Here's the drawing with two shaded views (mm, measured from the low corner). I have some questions. A direction names the side the tool comes from. Coordinates: 2 decimals unless noted, no trailing zeros. Write each loop counter-clockwise with the first axis right and the second up, starting at its lowest first coordinate (ties: lowest second). Pieces come first, ordered by that corner, then holes.
Item 1: If I drill on line 1 (Z direction, x = 100.5, y = 17.5); line 2 (Y direction, x = 9.5, z = 70), over which ranges is the centre line in solid material (lowest first)?
Item 2: For the marked faces 1 and 2, which set-ups out of +Z, -Z, +X, -X, +Y, -Y let a thin tool reach every point of the face, with its end or its side?
Item 3: If we section it at B-B (x = 35): Please give me the cut outline in (y, z).
Item 4: If we section it at C-C (z = 157.5): Please give me the cut outline in (x, y).
Item 5: If we section it at A-A (y = 26): Please give me the cut outline in (x, z), then the cut area to 3 significant figures.
Item 6: I'm going to push a flat-ended pin straight in: pin 1 Ø8 at (x, z) = (26, 38.5) entering from -Y. Where does the tip first touch, or does it pass through?
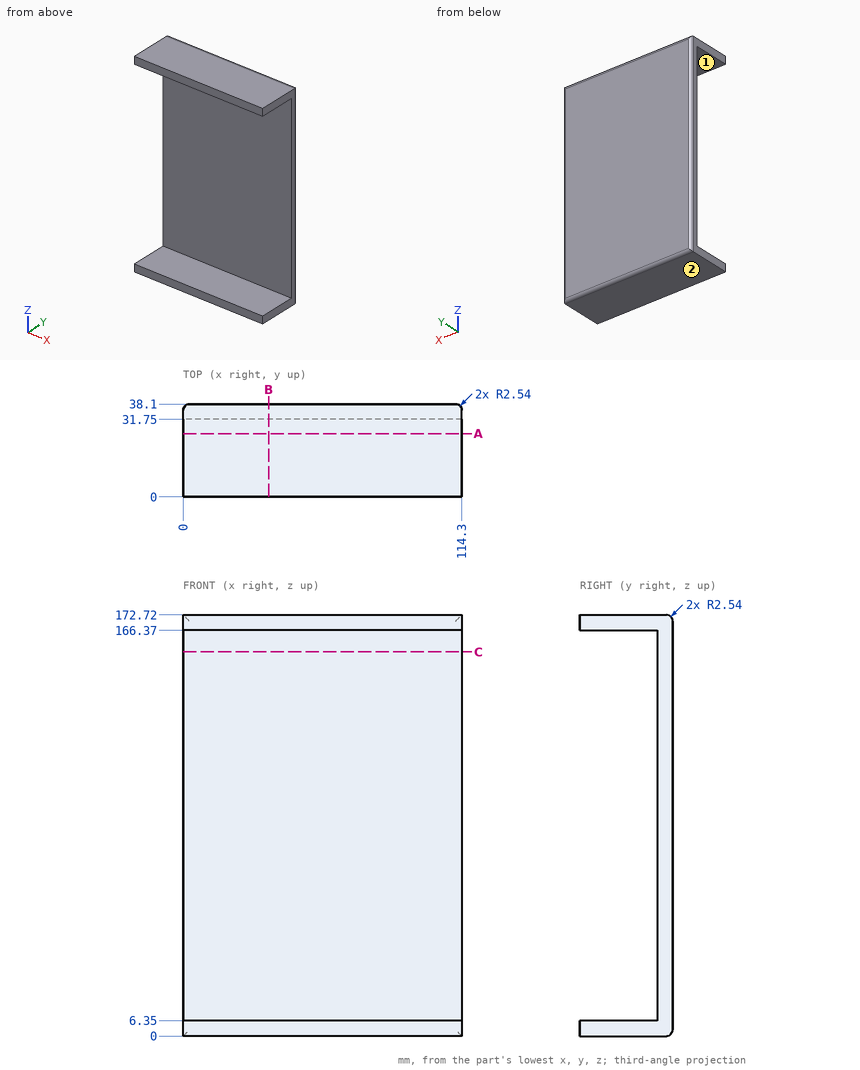
Answer list:
1. line 1: z = 0 to 6.35, 166.37 to 172.72
1. line 2: y = 31.75 to 38.1
2. face 1: +X, -X, -Y
2. face 2: -Z, +X, -X, +Y, -Y
3. outline: (0, 0) - (35.56, 0) arc R2.54 ccw to (38.1, 2.54) - (38.1, 170.18) arc R2.54 ccw to (35.56, 172.72) - (0, 172.72) - (0, 166.37) - (31.75, 166.37) - (31.75, 6.35) - (0, 6.35) - close
4. outline: (0, 31.75) - (114.3, 31.75) - (114.3, 35.56) arc R2.54 ccw to (111.76, 38.1) - (2.54, 38.1) arc R2.54 ccw to (0, 35.56) - close
5. outline: (0, 0) - (114.3, 0) - (114.3, 6.35) - (0, 6.35) - close; (0, 166.37) - (114.3, 166.37) - (114.3, 172.72) - (0, 172.72) - close
5. area: 1,450 mm2
6. pin 1: stops at y = 31.75
